```python
from build123d import *

# Parameters (mm, degrees)
F1_DEPTH    = 2.25
F2_R        = 10.6
F3_DEPTH    = 10.6
F5_DEPTH    = 9.5
F6_T2_ANGLE = 286.1981288485
F6_T4_ANGLE = 106.0815039342
F7_R        = 11.05
F8_DEPTH    = 10
F9_R        = 9
F10_DEPTH   = 7
F11_R       = 10.6
F11_R_2     = 9.6734059383
F12_DEPTH   = 8
F13_R       = 9.375
F14_DEPTH   = 1


# Not quite as in the source:
# - a fillet or chamfer that OpenCascade refuses, or shapes differently, is made with other operations: its cross-section is extruded or revolved along the edge and cut away or added


with BuildPart() as f1:
    # F0 (on Top) → F1 (new body)
    with BuildSketch(Plane.XY):
        Polygon((0, 11.1803398875), (10, 0), (23.8196601125, 0), (35, 10), (35, 25), (23.8196601125, 35), (10, 35), (0, 23.8196601125), align=None)
    extrude(amount=F1_DEPTH)

    # F2 (on Top) → F3 (join)
    with BuildSketch(Plane.XY):
        with Locations((17.5, 17.5)):
            Circle(F2_R)
    extrude(amount=F3_DEPTH)

    # F4 (on face) → F5 (join)
    with BuildSketch(Plane(origin=(0, 0, 0), x_dir=(1, 0, 0), z_dir=(0, 0, -1))):
        with BuildLine():
            ThreePointArc((11.9493243654, -6.3), (10.909607198, -28.1215216761), (30, -17.5))
            ThreePointArc((30, -17.5), (28.1215216761, -10.909607198), (23.0506756346, -6.3))
            Line((23.0506756346, -6.3), (11.9493243654, -6.3))
        make_face()
    extrude(amount=F5_DEPTH)

    # F6: chamfer of 1.5 on 2 edges, made by hand

    # F6_s1 → F6_t2 (revolve, cut)
    with BuildSketch(Plane(origin=(20.8261774668, 6.0498263405, 0), x_dir=(0, 0, 1), z_dir=(0.9603027964, 0.2789597449, 0))):
        with BuildLine():
            Line((-7.9575735931, 0.618923005), (-9.5424264069, -0.9659298087))
            Line((-9.5424264069, -0.9659298087), (-9.5724264069, -0.9659298087))
            ThreePointArc((-9.5724264069, -0.9659298087), (-9.53, -0.1947166053), (-9.53, 0.5764965982))
            Line((-9.53, 0.5764965982), (-9.5, 0.6064965982))
            ThreePointArc((-9.5, 0.6064965982), (-8.7287867966, 0.6064965982), (-7.9575735931, 0.648923005))
            Line((-7.9575735931, 0.648923005), (-7.9575735931, 0.618923005))
        make_face()
    revolve(axis=Axis((17.5, 17.5, -9.5), (0, 0, -1)), revolution_arc=F6_T2_ANGLE, mode=Mode.SUBTRACT)

    # F6_s3 → F6_t4 (revolve, cut)
    with BuildSketch(Plane.XZ.offset(-17.5)):
        with BuildLine():
            Line((30.0424264069, -7.9575735931), (28.4575735931, -9.5424264069))
            Line((28.4575735931, -9.5424264069), (28.4575735931, -9.5724264069))
            ThreePointArc((28.4575735931, -9.5724264069), (29.2287867966, -9.53), (30, -9.53))
            Line((30, -9.53), (30.03, -9.5))
            ThreePointArc((30.03, -9.5), (30.03, -8.7287867966), (30.0724264069, -7.9575735931))
            Line((30.0724264069, -7.9575735931), (30.0424264069, -7.9575735931))
        make_face()
    revolve(axis=Axis((17.5, 17.5, -9.5), (0, 0, -1)), revolution_arc=F6_T4_ANGLE, mode=Mode.SUBTRACT)

    # F7 (on face) → F8 (join)
    with BuildSketch(Plane(origin=(0, 0, -9.5), x_dir=(1, 0, 0), z_dir=(0, 0, -1))):
        with Locations((17.5, -17.5)):
            Circle(F7_R)
    extrude(amount=F8_DEPTH)

    # F9 (on face) → F10 (cut)
    with BuildSketch(Plane.XY.offset(10.6)):
        with Locations((17.5, 17.5)):
            Circle(F9_R)
    extrude(amount=-F10_DEPTH, mode=Mode.SUBTRACT)

    # F11 (on face) → F12 (cut)
    with BuildSketch(Plane.XY.offset(10.6)):
        with Locations((17.5, 17.5)):
            Circle(F11_R)
        with Locations((17.5, 17.5)):
            Circle(F11_R_2, mode=Mode.SUBTRACT)
    extrude(amount=-F12_DEPTH, mode=Mode.SUBTRACT)

    # F13 (on face) → F14 (cut)
    with BuildSketch(Plane(origin=(0, 0, -19.5), x_dir=(1, 0, 0), z_dir=(0, 0, -1))):
        with Locations((17.5, -17.5)):
            Circle(F13_R)
    extrude(amount=-F14_DEPTH, mode=Mode.SUBTRACT)


solid = f1.part
```
Read the model definition and answer for the solid it produces. Units are mm, in the model's axes. A direction names the side the tool comes from. Round coordinates to 2 decimals unless told otherwise and drop trailing zeros. Loops run counter-clockwise (first coordinate to the right, second up) from the corner with the lowest first, then second, coordinate; pieces in that order, holes last. Notation, with made-up numbers: (-17, -35) -> (-5, -35) arc R20 ccw to (-5, -18) -> close; hole circle Ø5 at (70.25, -4). An arc over 180 degrees is marked (long way). One line per item, written item: value.
1) The mould has two halves that part along Y. Classify faces 1 (the face through (29.49, 29.93, 1.11)), 2 (the face through (17, 0, 1)), 3 (the face through (17, 18, 3.6)): pulls with the +Y half, pulls with the -Y half, needs draft (parallel to the pull), parting line crosses it, or undercut.
Answer list:
face 1: pulls with the +Y half
face 2: pulls with the -Y half
face 3: undercut
2) A cutting plane is placed at B-B (z = 5.5). Determine the outline of the cut face in (x, y).
Answer list:
outline: circle Ø19.35 at (17.5, 17.5); hole circle Ø18 at (17.5, 17.5)
3) A cutting plane is placed at D-D (y = 5). Determine the outline of the cut face in (x, z), and give its area (3 significant figures).
Answer list:
outline: (5.53, 0) -> (29.41, 0) -> (29.41, 2.25) -> (5.53, 2.25) -> close
area: 53.7 mm²
4) A cutting plane is placed at C-C (z = -0.5). Determine the outline of the cut face in (x, y).
Answer list:
outline: (11.95, 6.3) -> (23.05, 6.3) arc R12.5 ccw (long way) to start
5) For faces 4 (the face through (27.29, 13.44, 2.42)), 5 (the face through (13, 26, -19.5)), 6 (the face through (26.44, 14.68, -19.01)), determine the directions among +Z, -Z, +X, -X, +Y, -Y from which every point of the face is accessible in a straight line to the end or side of a thin tool.
Answer list:
face 4: +Z
face 5: -Z, +X, -X, +Y, -Y
face 6: -Z
6) Flat-ended cylindrical pins translate along their axes: P1, Ø6, axis at y = 7, z = -12, coming from the +X side; P2, Ø5, axis at y = 12, z = 5.5, coming from the -X side; P3, Ø9.5, axis at x = 16.5, y = 20, coming from the -Z side. Find the tip coordinate at first contact, or state that the pin passes through.
Answer list:
P1: stops at x = 25.61
P2: stops at x = 8.3
P3: stops at z = -18.5
7) Consider L1, parallel to Y at x = 17.5, z = -18.65 (3 decimals); L2, parallel to X at y = 17, z = -18; L3, parallel to Y at x = 17.5, z = 9. Determine where each line is inside the solid, lowest interval first. Write a range as [from, to].
Answer list:
L1: y = [6.45, 8.125], [26.875, 28.55]
L2: x = [6.46, 28.54]
L3: y = [7.83, 8.5], [26.5, 27.17]
